Check sheet for the modelled part. Datum: model origin and axes. Units: mm. A direction names the side the tool comes from. Round coordinates to 2 decimals unless told otherwise and drop trailing zeros. Order: outer loops, then holes, each group sorted by start corner. A loop starts at its lowest first (then second) coordinate and runs counter-clockwise, first axis right, second up. Notation, with made-up numbers: M 50.5,26 L 75.5,26 A33 ccw 75.5,55 Z; hole C 36,-31.5 d11. An arc over 180 degrees is marked long. One line per item, written item: value. Start each with the question number.
(1) Access from +Z, -Z, +X, -X, +Y, -Y to the whole of each face (thin tool, end or side, straight path). Record for faces 1 (the face through (25, 86.085, 9)), 2 (the face through (0, 54, -6)), 3 (the face through (26, 93, 23.05)).
(2) Cross-section at B-B, the plane x = 37. Enter the section's corners in (y, z), and give its area (3 significant figures).
(3) Cross-section at C-C, the plane y = 21. Enter the section's corners in (x, z), and give its area (3 significant figures).
(4) Thickness scan on L1, parallel to Z at x = 27.5, y = 89.5; L2, parallel to Y at x = 22, z = 28.5; L3, parallel to X at y = 21.5, z = 11. Record the ranges inside material, lowest first.
(5) Release check for a two-part mould opening along Y. For faces 4 (the face through (25, 9.885, 5)), 5 (the face through (50.8, 54, -6)), 6 (the face through (25, 55, -2.35)), 7 (the face through (25, 22.585, 25)) record: released by +Y, released by -Y, zero draft, split by the parting line, or undercut.
(6) Cross-section at A-A, the plane z = 14. Enter the section's corners in (x, y), and give its area (3 significant figures).
(7) Depth check by flat-ended pin: pin 1 Ø2 at (x, y) = (27, 56.5) entering from +Z. Enter the tip coordinate at first touch or a pass-through.
(8) Cross-section at D-D, the plane z = 25. Enter the section's corners in (x, y), and give its area (3 significant figures).
from build123d import *

# Parameters (mm, degrees)
F1_DEPTH = 50.8
F2_W     = 25.4
F2_H     = 12.7
F3_DEPTH = 88.9


with BuildPart() as f1:
    # F0 (on Right) → F1 (new body)
    with BuildSketch(Plane.YZ):
        Polygon((98.784957, 35.750121), (86.084957, 35.750121), (86.084957, -2.349879), (22.584957, -2.349879), (22.584957, 35.750121), (9.884957, 35.750121), (9.884957, -15.049879), (22.584957, -15.049879), (86.084957, -15.049879), (98.784957, -15.049879), align=None)
    extrude(amount=F1_DEPTH)

    # F2 (on face) → F3 (cut)
    with BuildSketch(Plane(origin=(0, 98.784957, 0), x_dir=(-1, 0, 0), z_dir=(0, 1, 0))):
        with Locations((-25.4, 16.700121)):
            Rectangle(F2_W, F2_H)
    extrude(amount=-F3_DEPTH, mode=Mode.SUBTRACT)


solid = f1.part
Values found:
1. face 1: +Z, +X, -X
1. face 2: +Z, -Z, -X, +Y, -Y
1. face 3: +Y, -Y
2. outline: M 9.88,-15.05 L 98.78,-15.05 L 98.78,10.35 L 86.08,10.35 L 86.08,-2.35 L 22.58,-2.35 L 22.58,10.35 L 9.88,10.35 Z; M 9.88,23.05 L 22.58,23.05 L 22.58,35.75 L 9.88,35.75 Z; M 86.08,23.05 L 98.78,23.05 L 98.78,35.75 L 86.08,35.75 Z
2. area: 1,770 mm^2
3. outline: M 0,-15.05 L 50.8,-15.05 L 50.8,35.75 L 0,35.75 Z; hole M 12.7,10.35 L 38.1,10.35 L 38.1,23.05 L 12.7,23.05 Z
3. area: 2,260 mm^2
4. L1: -15.05 to 10.35, 23.05 to 35.75
4. L2: 9.88 to 22.58, 86.08 to 98.78
4. L3: 0 to 12.7, 38.1 to 50.8
5. face 4: released by -Y
5. face 5: zero draft
5. face 6: undercut
5. face 7: undercut
6. outline: M 0,9.88 L 12.7,9.88 L 12.7,22.58 L 0,22.58 Z; M 0,86.08 L 12.7,86.08 L 12.7,98.78 L 0,98.78 Z; M 38.1,9.88 L 50.8,9.88 L 50.8,22.58 L 38.1,22.58 Z; M 38.1,86.08 L 50.8,86.08 L 50.8,98.78 L 38.1,98.78 Z
6. area: 645 mm^2
7. pin 1: z = -2.35
8. outline: M 0,9.88 L 50.8,9.88 L 50.8,22.58 L 0,22.58 Z; M 0,86.08 L 50.8,86.08 L 50.8,98.78 L 0,98.78 Z
8. area: 1,290 mm^2
